Model file for the job. Use its own axes, mm. Give positions to 0.01 mm unless a question says otherwise; leave off trailing zeros. Loops run counter-clockwise (first coordinate to the right, second up) from the corner with the lowest first, then second, coordinate; pieces in that order, holes last. Notation, with made-up numbers: M 83,75 L 132,75 A21 cw 132,113 Z; hole C -2.75,83.25 d5. An arc over 180 degrees is marked long. Answer in a Markdown table with one row per item.
```python
from build123d import *

# Parameters (mm, degrees)
F0_R     = 41
F0_W     = 60
F0_H     = 3
F0_W_2   = 3
F0_H_2   = 60
F1_DEPTH = 3


with BuildPart() as f1:
    # F0 (on Top) → F1 (new body)
    with BuildSketch(Plane.XY):
        Polygon((72, 30), (72, 57), (30, 57), (-30, 57), (-72, 57), (-72, 30), (-72, -30), (-72, -57), (-30, -57), (30, -57), (72, -57), (72, -30), align=None)
        Circle(F0_R, mode=Mode.SUBTRACT)
        with Locations((0, 58.5)):
            Rectangle(F0_W, F0_H)
        with Locations((73.5, 0)):
            Rectangle(F0_W_2, F0_H_2)
        with Locations((-73.5, 0)):
            Rectangle(F0_W_2, F0_H_2)
        with Locations((0, -58.5)):
            Rectangle(F0_W, F0_H)
    extrude(amount=F1_DEPTH)


solid = f1.part
```
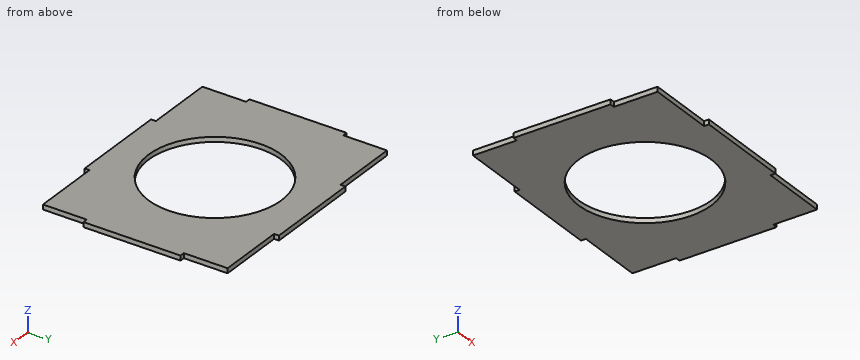
Q1. Drop flat-ended pins along their axis: pin 1 (1.5 mm diameter, centred on x = -48.5, z = 1.5, fed in from +Y); pin 2 (1.5 mm diameter, centred on y = -58.5, z = 2, fed in from -X); pin 3 (0.9 mm diameter, centred on y = 39, z = 1, fed in from +X). Give the stop position or say it passes through.
Reported:
| item | result |
|---|---|
| pin 1 | y = 57 |
| pin 2 | x = -30 |
| pin 3 | x = 72 |
Q2. Saw through at B-B (x = 0). Give the cut face in (y, z).
Reported:
| item | result |
|---|---|
| outline | M -60,0 L -41,0 L -41,3 L -60,3 Z; M 41,0 L 60,0 L 60,3 L 41,3 Z |
Q3. Saw through at D-D (x = 61). Give the cut face in (y, z).
Reported:
| item | result |
|---|---|
| outline | M -57,0 L 57,0 L 57,3 L -57,3 Z |
Q4. Probe probe 1 along Y at (x, z) = (0, 1.8); probe 2 along Y at (x, z) = (14.5, 2.4); probe 3 along X at (y, z) = (1.5, 2.7). List the from-to ranges inside material, lowest first.
Reported:
| item | result |
|---|---|
| probe 1 | -60 to -41, 41 to 60 |
| probe 2 | -60 to -38.35, 38.35 to 60 |
| probe 3 | -75 to -40.97, 40.97 to 75 |
Q5. Saw through at A-A (y = 0). Give the cut face in (x, z), and give its area (3 significant figures).
Reported:
| item | result |
|---|---|
| outline | M -75,0 L -41,0 L -41,3 L -75,3 Z; M 41,0 L 75,0 L 75,3 L 41,3 Z |
| area | 204 mm² |
Q6. Saw through at C-C (z = 0.45). Give the cut face in (x, y).
Reported:
| item | result |
|---|---|
| outline | M -75,-30 L -72,-30 L -72,-57 L -30,-57 L -30,-60 L 30,-60 L 30,-57 L 72,-57 L 72,-30 L 75,-30 L 75,30 L 72,30 L 72,57 L 30,57 L 30,60 L -30,60 L -30,57 L -72,57 L -72,30 L -75,30 Z; hole C 0,0 d82 |
